```python
from build123d import *

# Parameters (mm, degrees)
F0_R      = 19.558
F1_DEPTH  = 16.764
F2_R      = 8.509
F3_DEPTH  = 12.446
F4_R      = 18.034
F4_R_2    = 9.652
F5_DEPTH  = 15.24
F6_R      = 9.652
F7_DEPTH  = 2.032
F8_R      = 1.905
F9_DEPTH  = 25.4
F10_R     = 1.905
F11_DEPTH = 5.08
F10_R_2   = 3.7465
F12_DEPTH = 2.54
F13_R     = 0.381
F14_DEPTH = 0.508
F15_R     = 1.5875
F16_DEPTH = 5.8674


with BuildPart() as f1:
    # F0 (on Front) → F1 (new body)
    with BuildSketch(Plane.XZ):
        Circle(F0_R)
    extrude(amount=F1_DEPTH)

    # F2 (on face) → F3 (cut)
    with BuildSketch(Plane.XZ.offset(16.764)):
        Circle(F2_R)
    extrude(amount=-F3_DEPTH, mode=Mode.SUBTRACT)

    # F4 (on face) → F5 (cut)
    with BuildSketch(Plane(origin=(0, 0, 0), x_dir=(-1, 0, 0), z_dir=(0, 1, 0))):
        Circle(F4_R)
        Circle(F4_R_2, mode=Mode.SUBTRACT)
    extrude(amount=-F5_DEPTH, mode=Mode.SUBTRACT)

    # F6 (on face) → F7 (cut)
    with BuildSketch(Plane(origin=(0, 0, 0), x_dir=(-1, 0, 0), z_dir=(0, 1, 0))):
        Circle(F6_R)
    extrude(amount=-F7_DEPTH, mode=Mode.SUBTRACT)

    # F8 (on face) → F9 (cut)
    with BuildSketch(Plane(origin=(0, -2.032, 0), x_dir=(-1, 0, 0), z_dir=(0, 1, 0))):
        with Locations((4.22072, -4.22072)):
            Circle(F8_R)
        with Locations((5.969, 0)):
            Circle(F8_R)
        with Locations((4.22072, 4.22072)):
            Circle(F8_R)
        with Locations((0, 5.969)):
            Circle(F8_R)
        with Locations((-4.22072, 4.22072)):
            Circle(F8_R)
        with Locations((-5.969, 0)):
            Circle(F8_R)
        with Locations((-4.22072, -4.22072)):
            Circle(F8_R)
        with Locations((0, -5.969)):
            Circle(F8_R)
    extrude(amount=-F9_DEPTH, mode=Mode.SUBTRACT)

    # F10 (on face) → F11 (join)
    with BuildSketch(Plane.XZ.offset(4.318)):
        Circle(F10_R)
    extrude(amount=F11_DEPTH)

    # F10 (on face) → F12 (join)
    with BuildSketch(Plane.XZ.offset(4.318)):
        Circle(F10_R_2)
        Circle(F10_R, mode=Mode.SUBTRACT)
    extrude(amount=F12_DEPTH)

    # F13 (on face) → F14 (join)
    with BuildSketch(Plane.XZ.offset(6.858)):
        with Locations((0, 2.82575)):
            Circle(F13_R)
        with Locations((-1.660934, 2.28608)):
            Circle(F13_R)
        with Locations((-2.687448, 0.873205)):
            Circle(F13_R)
        with Locations((-2.687448, -0.873205)):
            Circle(F13_R)
        with Locations((-1.660934, -2.28608)):
            Circle(F13_R)
        with Locations((0, -2.82575)):
            Circle(F13_R)
        with Locations((1.660934, -2.28608)):
            Circle(F13_R)
        with Locations((2.687448, -0.873205)):
            Circle(F13_R)
        with Locations((2.687448, 0.873205)):
            Circle(F13_R)
        with Locations((1.660934, 2.28608)):
            Circle(F13_R)
    extrude(amount=F14_DEPTH)

    # F15 (on face) → F16 (cut)
    with BuildSketch(Plane(origin=(0, -2.032, 0), x_dir=(-1, 0, 0), z_dir=(0, 1, 0))):
        Circle(F15_R)
    extrude(amount=-F16_DEPTH, mode=Mode.SUBTRACT)


solid = f1.part
```
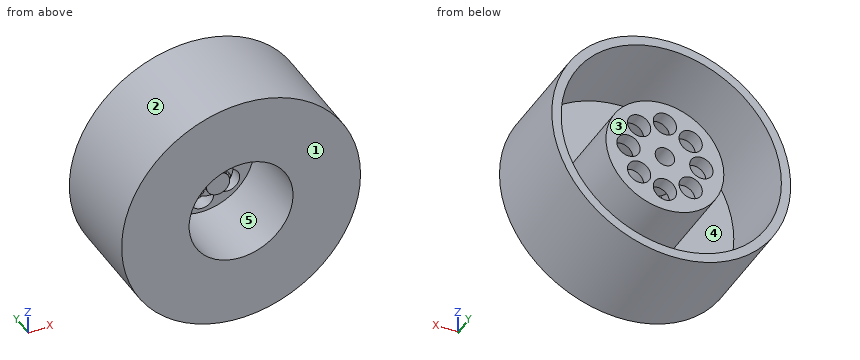
Here's how the part is built. I have some questions about the finished solid (model axes, mm). Face numbers are marked on the shaded views. A direction names the side the tool comes from. Coordinates: 2 decimals unless noted, no trailing zeros. Order: outer loops, then holes, each group sorted by start corner. A loop starts at its lowest first (then second) coordinate and runs counter-clockwise, first axis right, second up. Notation, with made-up numbers: (-4.75, 44) -> (43.25, 44) arc R31 ccw to (43.25, 80) -> close; hole circle Ø3 at (66, 43). An arc over 180 degrees is marked (long way). Return JSON: item names as keys, results as strings.
1) On a 3-axis mill with a long thin cutter (end or side, diameter ignored), from which of +Z, -Z, +X, -X, +Y, -Y can I reach the whole of each face in a straight line? I mean the marked faces 4 and 5. Say none if no direction works.
Conclusion:
{"face 4": "+Y", "face 5": "-Y"}
2) If I drill on probe 1 along Z at (x, y) = (0, -3.25); probe 2 along X at (y, z) = (-5.75, 4); probe 3 along X at (y, z) = (-9, 2.5), over which ranges is the centre line in solid material (lowest first)?
Conclusion:
{"probe 1": "z = -19.56 to -18.03, -9.65 to -7.87, -4.06 to -1.59, 1.59 to 4.06, 7.87 to 9.65, 18.03 to 19.56", "probe 2": "x = -19.14 to -17.58, -8.78 to -7.51, 7.51 to 8.78, 17.58 to 19.14", "probe 3": "x = -19.4 to -17.86, -9.32 to -8.13, 8.13 to 9.32, 17.86 to 19.4"}
3) If we section it at D-D on y = -3: State how many separate pieces and enclosed holes the cut face has, plus the area to 3 significant figures.
Conclusion:
{"separate pieces": "2", "enclosed holes": "10", "area": "374 mm²"}
4) If we section it at C-C on x = 5.5: List the corners of the cut face in (y, z) for me.
Conclusion:
{"outline": "(-16.76, -18.77) -> (0, -18.77) -> (0, -17.17) -> (-15.24, -17.17) -> (-15.24, -7.93) -> (-2.03, -7.93) -> (-2.03, -5.63) -> (-4.32, -5.63) -> (-4.32, -6.49) -> (-16.76, -6.49) -> close; (-16.76, 6.49) -> (-4.32, 6.49) -> (-4.32, 5.63) -> (-2.03, 5.63) -> (-2.03, 7.93) -> (-15.24, 7.93) -> (-15.24, 17.17) -> (0, 17.17) -> (0, 18.77) -> (-16.76, 18.77) -> close; (-4.32, -2.81) -> (-2.03, -2.81) -> (-2.03, -1.85) -> (-4.32, -1.85) -> close; (-4.32, 1.85) -> (-2.03, 1.85) -> (-2.03, 2.81) -> (-4.32, 2.81) -> close"}
5) I'm going to push flat-ended pins straight in: P1, Ø3, axis at x = -4.22, z = -4.22, coming from the -Y side; P2, Ø5, axis at x = -7.5, y = -10, coming from the +Z side; P3, Ø1, axis at x = 5.5, z = 6, coming from the +Y side; P4, Ø6, axis at x = -1, y = -11.5, coming from the +Z side. Where does each tip first touch, or does it pass through?
Conclusion:
{"P1": "passes through", "P2": "stops at z = 18.91", "P3": "stops at y = -2.03", "P4": "stops at z = 19.56"}
6) If we section it at A-A on y = -8.5: List the corners of the cut face in (x, z) for me (3 decimals).
Conclusion:
{"outline": "circle Ø39.116 at (0, 0); circle Ø19.304 at (0, 0); circle Ø3.81 at (0, 0); hole circle Ø36.068 at (0, 0); hole circle Ø17.018 at (0, 0)"}
7) Thinking about a two-plate mould opening in Z: for the marked faces 1, 2 and 3, which applies, +Z half, -Z half, draft (parallel to the pull), parting line (faces both ways), or undercut?
Conclusion:
{"face 1": "draft", "face 2": "parting line", "face 3": "undercut"}
8) If we section it at B-B on y = -5.75: List the corners of the cut face in (x, z) for me (1 decimal).
Conclusion:
{"outline": "circle Ø39.1 at (0, 0); circle Ø19.3 at (0, 0); circle Ø7.5 at (0, 0); hole circle Ø36.1 at (0, 0); hole circle Ø17 at (0, 0); hole circle Ø3.2 at (0, 0)"}
